Work out the finished part from the listing and answer in its coordinate system (mm). Round coordinates to 2 decimals unless told otherwise and drop trailing zeros. Order: outer loops, then holes, each group sorted by start corner. A loop starts at its lowest first (then second) coordinate and runs counter-clockwise, first axis right, second up. Notation, with made-up numbers: M 7,64 L 39,64 A23 cw 39,97 Z; hole C 44,71.25 d5. An arc over 180 degrees is marked long. Answer as a JSON object with one key per item and string values. Group by question number.
Autodesk Inventor part; units mm, degrees
ref_plane "YZ Plane" through (0, 0, 0) normal (1, 0, 0) x (0, 1, 0)
ref_plane "XZ Plane" through (0, 0, 0) normal (0, 1, 0) x (-1, 0, 0)
ref_plane "XY Plane" through (0, 0, 0) normal (0, 0, 1) x (1, 0, 0)
sketch "Sketch1" plane through (0, 0, 0) normal (0, 1, 0) x (-1, 0, 0)
  line L0 (0, 0) -> (380, 0)
  line L1 (380, 0) -> (380, -430)
  line L2 (380, -430) -> (0, -430)
  line L3 (0, -430) -> (0, 0)
  dimension "d0" = 380
  dimension "d1" = 430
extrude "Extrusion1" add sketch "Sketch1" along normal blind 50.8
sketch "Sketch2" plane through (0, 50.8, 0) normal (0, 1, 0) x (1, 0, 0)
  circle A0 centre (-220, 215) radius 5
  line L0 (0, 430) -> (-380, 430)
  line L1 (0, 0) -> (0, 430)
  line L2 (-380, 430) -> (-380, 0)
  dimension "d4" = 10
  dimension "d10" = 215
  dimension "d11" = 160
extrude "Extrusion2" cut sketch "Sketch2" against normal blind 50.8
sketch "Sketch3" plane through (0, 50.8, 0) normal (0, 1, 0) x (1, 0, 0)
  circle A0 centre (-170, 130) radius 5
  line L0 (0, 0) -> (0, 430)
  line L1 (-380, 0) -> (0, 0)
  circle A1 centre (-190, 130) radius 5
  circle A2 centre (-210, 130) radius 5
  circle A3 centre (-230, 130) radius 5
  dimension "d12" = 10
  dimension "d13" = 170
  dimension "d14" = 130
  dimension "d20" = 20
extrude "Extrusion3" cut sketch "Sketch3" against normal blind 50.8
sketch "Sketch4" plane through (0, 50.8, 0) normal (0, 1, 0) x (1, 0, 0)
  circle A0 centre (-170, 300) radius 5
  line L0 (0, 0) -> (0, 430)
  line L1 (0, 430) -> (-380, 430)
  circle A1 centre (-190, 300) radius 5
  circle A2 centre (-210, 300) radius 5
  circle A3 centre (-230, 300) radius 5
  dimension "d24" = 10
  dimension "d25" = 170
  dimension "d26" = 130
  dimension "d32" = 20
extrude "Extrusion4" cut sketch "Sketch4" against normal blind 50.8
sketch "Sketch5" plane through (0, 50.8, 0) normal (0, 1, 0) x (1, 0, 0)
  circle A0 centre (-260, 170) radius 5
  line L0 (-380, 430) -> (-380, 0)
  line L1 (-380, 0) -> (0, 0)
  circle A1 centre (-140, 170) radius 5
  line L2 (0, 0) -> (0, 430)
  circle A2 centre (-260, 200) radius 5
  circle A3 centre (-140, 200) radius 5
  circle A4 centre (-260, 230) radius 5
  circle A5 centre (-140, 230) radius 5
  circle A6 centre (-260, 260) radius 5
  circle A7 centre (-140, 260) radius 5
  dimension "d36" = 10
  dimension "d37" = 120
  dimension "d38" = 170
  dimension "d39" = 10
  dimension "d40" = 170
  dimension "d41" = 140
  dimension "d47" = 30
extrude "Extrusion5" cut sketch "Sketch5" against normal blind 50.8
properties part number "Trasera"
Item 1: Find section B-B (x = -260). Give the vertices of the cut face in (y, z), and give its area (3 significant figures).
Item 2: Find section A-A (z = -130). Give the vertices of the cut face in (x, y).
Item 3: The mould has two halves that part along Z. Classify faces 1 (the flat face through (-187, 50.8, -212)), 2 (the cylindrical face through (-140.651, 25.756, -234.957)), 3 (the cylindrical face through (-255.23, 25.76, -201.5)), 4 (the flat face through (-187, 25, 0)): +Z half, -Z half, draft (parallel to the pull), parting line (faces both ways), or undercut.
Item 4: This flat-tipped pin is pushed along its axis until it touches: pin 1 (6 mm diameter, centred on x = -190, z = -300, fed in from -Y). Where does it stop, or does it pass through?
Item 5: Find section C-C (z = -260). Give the vertices of the cut face in (x, y), and give its area (3 significant figures).
Item 6: Consider L1, parallel to Z at x = -260, y = 22; L2, parallel to X at y = 21, z = -230; L3, parallel to X at y = 40.5, z = -300. Determine where each line is inside the solid, lowest interval first.
Responses:
{
 "1": {"outline": "M 0,-430 L 50.8,-430 L 50.8,-265 L 0,-265 Z; M 0,-255 L 50.8,-255 L 50.8,-235 L 0,-235 Z; M 0,-225 L 50.8,-225 L 50.8,-205 L 0,-205 Z; M 0,-195 L 50.8,-195 L 50.8,-175 L 0,-175 Z; M 0,-165 L 50.8,-165 L 50.8,0 L 0,0 Z", "area": "19,800 mm^2"},
 "2": {"outline": "M -380,0 L -235,0 L -235,50.8 L -380,50.8 Z; M -225,0 L -215,0 L -215,50.8 L -225,50.8 Z; M -205,0 L -195,0 L -195,50.8 L -205,50.8 Z; M -185,0 L -175,0 L -175,50.8 L -185,50.8 Z; M -165,0 L 0,0 L 0,50.8 L -165,50.8 Z"},
 "3": {"face 1": "draft", "face 2": "undercut", "face 3": "undercut", "face 4": "+Z half"},
 "4": {"pin 1": "passes through"},
 "5": {"outline": "M -380,0 L -265,0 L -265,50.8 L -380,50.8 Z; M -255,0 L -145,0 L -145,50.8 L -255,50.8 Z; M -135,0 L 0,0 L 0,50.8 L -135,50.8 Z", "area": "18,300 mm^2"},
 "6": {"L1": "z = -430 to -265, -255 to -235, -225 to -205, -195 to -175, -165 to 0", "L2": "x = -380 to -265, -255 to -145, -135 to 0", "L3": "x = -380 to -235, -225 to -215, -205 to -195, -185 to -175, -165 to 0"}
}
